Can you work these out from the drawing? Everything is in mm from the part's minimum corner. A direction names the side the tool comes from. Give positions to 0.01 mm unless a question says otherwise; leave off trailing zeros. Order: outer loops, then holes, each group sorted by start corner. A loop starts at its lowest first (then second) coordinate and runs counter-clockwise, first axis right, second up. Notation, with made-up numbers: (23, -12.75) - (70, -12.75) arc R30 ccw to (70, 23.25) - close; hole circle Ø2 at (-4, 78). An arc over 180 degrees is marked (long way). One line per question, with ' | ' between items.
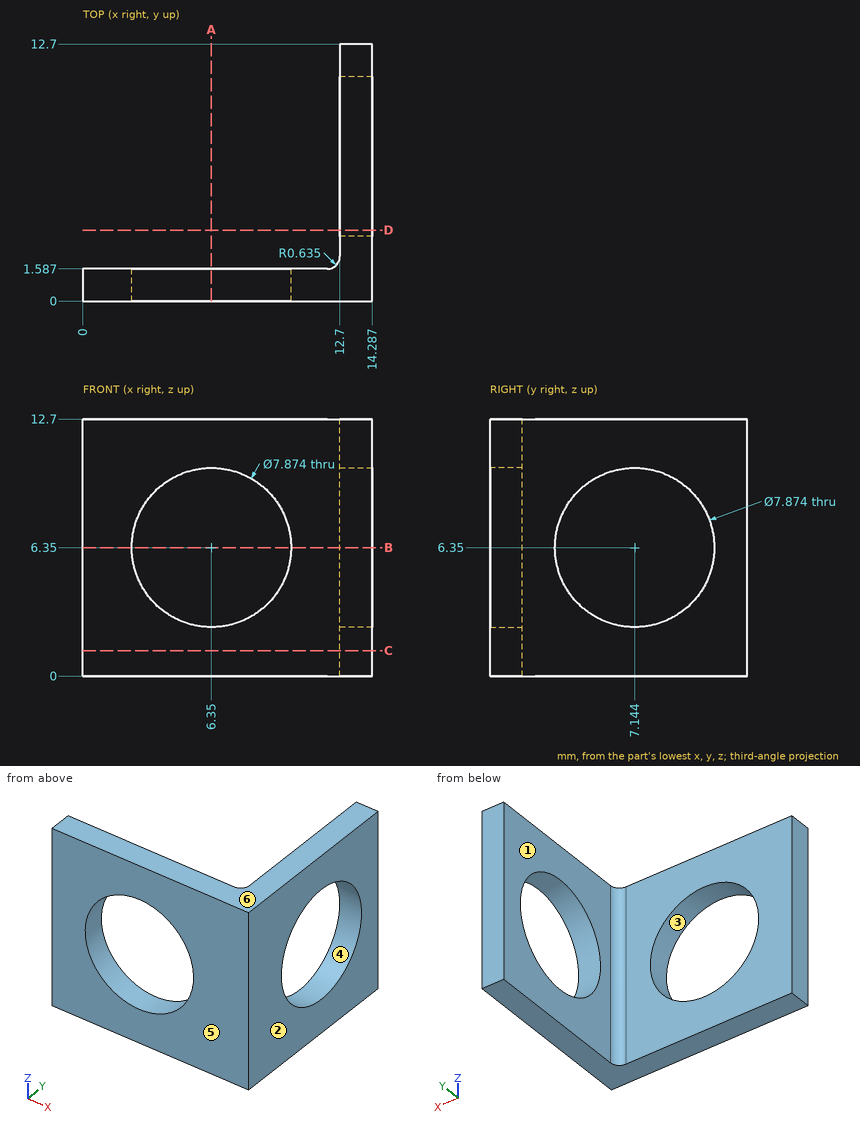
(1) If I drill on line 1 (Y direction, x = 13.2, z = 6.35); line 2 (X direction, y = 1.25, z = 6.35); line 3 (X direction, y = 3.25, z = 5.5), over which ranges is the centre line in solid material (lowest first)?
Answer below:
line 1: 0 to 3.21, 11.08 to 12.7 | line 2: 0 to 2.41, 10.29 to 14.29 | line 3: 12.7 to 14.29
(2) Imagine slicing it at D-D (y = 3.5). List the corners of the cut face in (x, z) for me.
Answer below:
outline: (12.7, 0) - (14.29, 0) - (14.29, 4.86) - (12.7, 4.86) - close; (12.7, 7.84) - (14.29, 7.84) - (14.29, 12.7) - (12.7, 12.7) - close
(3) Will these pins go through, and if not, where does the flat tip stop? pin 1 (2 mm diameter, centred on y = 6.5, z = 11, fed in from -X); pin 2 (3.5 mm diameter, centred on x = 8.5, z = 5, fed in from +Y); pin 3 (4 mm diameter, centred on x = 12.5, y = 2, fed in from -Z).
Answer below:
pin 1: x = 12.7 | pin 2: y = 1.59 | pin 3: z = 0
(4) On a 3-axis mill with a long thin cutter (end or side, diameter ignored), from which of +Z, -Z, +X, -X, +Y, -Y can I reach the whole of each face in a straight line? I mean the marked faces 1 and 2. Say none if no direction works.
Answer below:
face 1: +Z, -Z, -X, +Y | face 2: +Z, -Z, +X, +Y, -Y
(5) Imagine slicing it at A-A (x = 6.35). List the corners of the cut face in (y, z) for me.
Answer below:
outline: (0, 0) - (1.59, 0) - (1.59, 2.41) - (0, 2.41) - close; (0, 10.29) - (1.59, 10.29) - (1.59, 12.7) - (0, 12.7) - close
(6) Imagine slicing it at C-C (z = 1.25). List the corners of the cut face in (x, y) for me (1 decimal).
Answer below:
outline: (0, 0) - (14.3, 0) - (14.3, 12.7) - (12.7, 12.7) - (12.7, 2.2) arc R0.6 cw to (12.1, 1.6) - (0, 1.6) - close
(7) If we mould it in two halves opening along Z, with no side actions, what happens to the marked faces 3, 4, 5 and 6? For each: released by +Z, released by -Z, zero draft, split by the parting line, or undercut.
Answer below:
face 3: undercut | face 4: undercut | face 5: zero draft | face 6: released by +Z
(8) Imagine slicing it at B-B (z = 6.35). List the corners of the cut face in (x, y) for me (1 decimal), and give its area (3 significant figures).
Answer below:
outline: (0, 0) - (2.4, 0) - (2.4, 1.6) - (0, 1.6) - close; (10.3, 0) - (14.3, 0) - (14.3, 3.2) - (12.7, 3.2) - (12.7, 2.2) arc R0.6 cw to (12.1, 1.6) - (10.3, 1.6) - close; (12.7, 11.1) - (14.3, 11.1) - (14.3, 12.7) - (12.7, 12.7) - close | area: 15.4 mm^2
